```python
from build123d import *

# Parameters (mm, degrees)
BOSS_EXTRUDE2_DEPTH      = 1
SKETCH5_R                = 0.7
CUT_EXTRUDE2_DEPTH       = 1
LPATTERN2_COUNT          = 18
LPATTERN2_PITCH          = 2.47
MIRROR1_COPY_1_SKETCH_R  = 0.7
MIRROR1_COPY_1_DEPTH     = 1
MIRROR1_COPY_2_SKETCH_R  = 0.7
MIRROR1_COPY_2_DEPTH     = 1
MIRROR1_COPY_3_SKETCH_R  = 0.7
MIRROR1_COPY_3_DEPTH     = 1
MIRROR1_COPY_4_SKETCH_R  = 0.7
MIRROR1_COPY_4_DEPTH     = 1
MIRROR1_COPY_5_SKETCH_R  = 0.7
MIRROR1_COPY_5_DEPTH     = 1
MIRROR1_COPY_6_SKETCH_R  = 0.7
MIRROR1_COPY_6_DEPTH     = 1
MIRROR1_COPY_7_SKETCH_R  = 0.7
MIRROR1_COPY_7_DEPTH     = 1
MIRROR1_COPY_8_SKETCH_R  = 0.7
MIRROR1_COPY_8_DEPTH     = 1
MIRROR1_COPY_9_SKETCH_R  = 0.7
MIRROR1_COPY_9_DEPTH     = 1
MIRROR1_COPY_10_SKETCH_R = 0.7
MIRROR1_COPY_10_DEPTH    = 1
MIRROR1_COPY_11_SKETCH_R = 0.7
MIRROR1_COPY_11_DEPTH    = 1
MIRROR1_COPY_12_SKETCH_R = 0.7
MIRROR1_COPY_12_DEPTH    = 1
MIRROR1_COPY_13_SKETCH_R = 0.7
MIRROR1_COPY_13_DEPTH    = 1
MIRROR1_COPY_14_SKETCH_R = 0.7
MIRROR1_COPY_14_DEPTH    = 1
MIRROR1_COPY_15_SKETCH_R = 0.7
MIRROR1_COPY_15_DEPTH    = 1
MIRROR1_COPY_16_SKETCH_R = 0.7
MIRROR1_COPY_16_DEPTH    = 1
MIRROR1_COPY_17_SKETCH_R = 0.7
MIRROR1_COPY_17_DEPTH    = 1
SKETCH6_W                = 27.254379167
SKETCH6_H                = 15.23216969
BOSS_EXTRUDE3_DEPTH      = 4


with BuildPart() as part:
    # Sketch4 → Boss-Extrude2 (new body)
    with BuildSketch(Plane(origin=(0, 0, 0), x_dir=(1, 0, 0), z_dir=(0, 1, 0))):
        Polygon((-23, -10), (23, -10), (23, -8), (27, -8), (27, 8), (23, 8), (23, 10), (-23, 10), align=None)
    extrude(amount=BOSS_EXTRUDE2_DEPTH)

    # Sketch5 → Cut-Extrude2 (cut)
    with BuildSketch(Plane(origin=(0, 1, 0), x_dir=(1, 0, 0), z_dir=(0, 1, 0))):
        with Locations((-21, 10)):
            Circle(SKETCH5_R)
    cut_extrude2 = extrude(amount=-CUT_EXTRUDE2_DEPTH, mode=Mode.SUBTRACT)

    # LPattern2: Cut-Extrude2 ×18
    with Locations(*[(i * LPATTERN2_PITCH, 0, 0) for i in range(1, LPATTERN2_COUNT)]):
        add(cut_extrude2, mode=Mode.SUBTRACT)

    # Mirror1: Cut-Extrude2 across plane
    add(cut_extrude2.mirror(Plane.XY), mode=Mode.SUBTRACT)

    # Mirror1 copy 1 sketch → Mirror1 copy 1 (cut)
    with BuildSketch(Plane(origin=(2.47, 1, 0), x_dir=(1, 0, 0), z_dir=(0, 1, 0))):
        with Locations((-21, -10)):
            Circle(MIRROR1_COPY_1_SKETCH_R)
    extrude(amount=-MIRROR1_COPY_1_DEPTH, mode=Mode.SUBTRACT)

    # Mirror1 copy 2 sketch → Mirror1 copy 2 (cut)
    with BuildSketch(Plane(origin=(4.94, 1, 0), x_dir=(1, 0, 0), z_dir=(0, 1, 0))):
        with Locations((-21, -10)):
            Circle(MIRROR1_COPY_2_SKETCH_R)
    extrude(amount=-MIRROR1_COPY_2_DEPTH, mode=Mode.SUBTRACT)

    # Mirror1 copy 3 sketch → Mirror1 copy 3 (cut)
    with BuildSketch(Plane(origin=(7.41, 1, 0), x_dir=(1, 0, 0), z_dir=(0, 1, 0))):
        with Locations((-21, -10)):
            Circle(MIRROR1_COPY_3_SKETCH_R)
    extrude(amount=-MIRROR1_COPY_3_DEPTH, mode=Mode.SUBTRACT)

    # Mirror1 copy 4 sketch → Mirror1 copy 4 (cut)
    with BuildSketch(Plane(origin=(9.88, 1, 0), x_dir=(1, 0, 0), z_dir=(0, 1, 0))):
        with Locations((-21, -10)):
            Circle(MIRROR1_COPY_4_SKETCH_R)
    extrude(amount=-MIRROR1_COPY_4_DEPTH, mode=Mode.SUBTRACT)

    # Mirror1 copy 5 sketch → Mirror1 copy 5 (cut)
    with BuildSketch(Plane(origin=(12.35, 1, 0), x_dir=(1, 0, 0), z_dir=(0, 1, 0))):
        with Locations((-21, -10)):
            Circle(MIRROR1_COPY_5_SKETCH_R)
    extrude(amount=-MIRROR1_COPY_5_DEPTH, mode=Mode.SUBTRACT)

    # Mirror1 copy 6 sketch → Mirror1 copy 6 (cut)
    with BuildSketch(Plane(origin=(14.82, 1, 0), x_dir=(1, 0, 0), z_dir=(0, 1, 0))):
        with Locations((-21, -10)):
            Circle(MIRROR1_COPY_6_SKETCH_R)
    extrude(amount=-MIRROR1_COPY_6_DEPTH, mode=Mode.SUBTRACT)

    # Mirror1 copy 7 sketch → Mirror1 copy 7 (cut)
    with BuildSketch(Plane(origin=(17.29, 1, 0), x_dir=(1, 0, 0), z_dir=(0, 1, 0))):
        with Locations((-21, -10)):
            Circle(MIRROR1_COPY_7_SKETCH_R)
    extrude(amount=-MIRROR1_COPY_7_DEPTH, mode=Mode.SUBTRACT)

    # Mirror1 copy 8 sketch → Mirror1 copy 8 (cut)
    with BuildSketch(Plane(origin=(19.76, 1, 0), x_dir=(1, 0, 0), z_dir=(0, 1, 0))):
        with Locations((-21, -10)):
            Circle(MIRROR1_COPY_8_SKETCH_R)
    extrude(amount=-MIRROR1_COPY_8_DEPTH, mode=Mode.SUBTRACT)

    # Mirror1 copy 9 sketch → Mirror1 copy 9 (cut)
    with BuildSketch(Plane(origin=(22.23, 1, 0), x_dir=(1, 0, 0), z_dir=(0, 1, 0))):
        with Locations((-21, -10)):
            Circle(MIRROR1_COPY_9_SKETCH_R)
    extrude(amount=-MIRROR1_COPY_9_DEPTH, mode=Mode.SUBTRACT)

    # Mirror1 copy 10 sketch → Mirror1 copy 10 (cut)
    with BuildSketch(Plane(origin=(24.7, 1, 0), x_dir=(1, 0, 0), z_dir=(0, 1, 0))):
        with Locations((-21, -10)):
            Circle(MIRROR1_COPY_10_SKETCH_R)
    extrude(amount=-MIRROR1_COPY_10_DEPTH, mode=Mode.SUBTRACT)

    # Mirror1 copy 11 sketch → Mirror1 copy 11 (cut)
    with BuildSketch(Plane(origin=(27.17, 1, 0), x_dir=(1, 0, 0), z_dir=(0, 1, 0))):
        with Locations((-21, -10)):
            Circle(MIRROR1_COPY_11_SKETCH_R)
    extrude(amount=-MIRROR1_COPY_11_DEPTH, mode=Mode.SUBTRACT)

    # Mirror1 copy 12 sketch → Mirror1 copy 12 (cut)
    with BuildSketch(Plane(origin=(29.64, 1, 0), x_dir=(1, 0, 0), z_dir=(0, 1, 0))):
        with Locations((-21, -10)):
            Circle(MIRROR1_COPY_12_SKETCH_R)
    extrude(amount=-MIRROR1_COPY_12_DEPTH, mode=Mode.SUBTRACT)

    # Mirror1 copy 13 sketch → Mirror1 copy 13 (cut)
    with BuildSketch(Plane(origin=(32.11, 1, 0), x_dir=(1, 0, 0), z_dir=(0, 1, 0))):
        with Locations((-21, -10)):
            Circle(MIRROR1_COPY_13_SKETCH_R)
    extrude(amount=-MIRROR1_COPY_13_DEPTH, mode=Mode.SUBTRACT)

    # Mirror1 copy 14 sketch → Mirror1 copy 14 (cut)
    with BuildSketch(Plane(origin=(34.58, 1, 0), x_dir=(1, 0, 0), z_dir=(0, 1, 0))):
        with Locations((-21, -10)):
            Circle(MIRROR1_COPY_14_SKETCH_R)
    extrude(amount=-MIRROR1_COPY_14_DEPTH, mode=Mode.SUBTRACT)

    # Mirror1 copy 15 sketch → Mirror1 copy 15 (cut)
    with BuildSketch(Plane(origin=(37.05, 1, 0), x_dir=(1, 0, 0), z_dir=(0, 1, 0))):
        with Locations((-21, -10)):
            Circle(MIRROR1_COPY_15_SKETCH_R)
    extrude(amount=-MIRROR1_COPY_15_DEPTH, mode=Mode.SUBTRACT)

    # Mirror1 copy 16 sketch → Mirror1 copy 16 (cut)
    with BuildSketch(Plane(origin=(39.52, 1, 0), x_dir=(1, 0, 0), z_dir=(0, 1, 0))):
        with Locations((-21, -10)):
            Circle(MIRROR1_COPY_16_SKETCH_R)
    extrude(amount=-MIRROR1_COPY_16_DEPTH, mode=Mode.SUBTRACT)

    # Mirror1 copy 17 sketch → Mirror1 copy 17 (cut)
    with BuildSketch(Plane(origin=(41.99, 1, 0), x_dir=(1, 0, 0), z_dir=(0, 1, 0))):
        with Locations((-21, -10)):
            Circle(MIRROR1_COPY_17_SKETCH_R)
    extrude(amount=-MIRROR1_COPY_17_DEPTH, mode=Mode.SUBTRACT)

    # Sketch6 → Boss-Extrude3 (add)
    with BuildSketch(Plane(origin=(0, 1, 0), x_dir=(1, 0, 0), z_dir=(0, 1, 0))):
        with Locations((-8.447512014, 0)):
            Rectangle(SKETCH6_W, SKETCH6_H)
    extrude(amount=BOSS_EXTRUDE3_DEPTH)


solid = part.part
```
Verification items for the finished model (mm, model axes). A direction names the side the tool comes from. Coordinates: 2 decimals unless noted, no trailing zeros. Write each loop counter-clockwise with the first axis right and the second up, starting at its lowest first coordinate (ties: lowest second). Pieces come first, ordered by that corner, then holes. Notation, with made-up numbers: (71, 61.5) - (128, 61.5) arc R19 cw to (128, 72.5) - close; hole circle Ø4 at (-15.5, 47.25). An arc over 180 degrees is marked (long way). Write item = value, one per line.
Q1. Cross-section at D-D (x = 13.58). Enter the section's corners in (y, z).
Answer:
outline = (0, -9.3) - (1, -9.3) - (1, 9.3) - (0, 9.3) - close
Q2. Material ranges on L1, parallel to Y at x = 20.5, z = 9; L2, parallel to X at y = 2.25, z = -1; L3, parallel to Z at x = -1, y = 2.35, recorded low to high. Write a range as from..to.
Answer:
L1 = 0..1
L2 = -22.07..5.18
L3 = -7.62..7.62
Q3. Cross-section at A-A (z = 5.5). Enter the section's corners in (x, y).
Answer:
outline = (-23, 0) - (27, 0) - (27, 1) - (5.18, 1) - (5.18, 5) - (-22.07, 5) - (-22.07, 1) - (-23, 1) - close
Q4. Mould release check, pull along X, two halves, no side actions. Record for faces 4 (the face through (13.6, 0.5, -9.3)), 5 (the face through (0, 0.5, 10)), 6 (the face through (23, 0.5, -9)), 7 (the face through (16.1, 0.5, 9.3)): released by +X, released by -X, zero draft, split by the parting line, or undercut.
Answer:
face_4 = undercut
face_5 = zero draft
face_6 = released by +X
face_7 = undercut
Q5. Cross-section at C-C (y = 2.85). Enter the section's corners in (x, z).
Answer:
outline = (-22.07, -7.62) - (5.18, -7.62) - (5.18, 7.62) - (-22.07, 7.62) - close
Q6. Cross-section at B-B (x = -21). Enter the section's corners in (y, z).
Answer:
outline = (0, -9.3) - (1, -9.3) - (1, -7.62) - (5, -7.62) - (5, 7.62) - (1, 7.62) - (1, 9.3) - (0, 9.3) - close
Q7. Access from +Z, -Z, +X, -X, +Y, -Y to the whole of each face (thin tool, end or side, straight path). Record for faces 1 (the face through (-9, 3, -7.616)), 2 (the face through (-9, 3, 7.616)), 3 (the face through (17.3, 0.5, -10)).
Answer:
face_1 = -Z, +X, -X, +Y
face_2 = +Z, +X, -X, +Y
face_3 = -Z, +X, -X, +Y, -Y
Q8. Go/stop test with flat-tipped pins: pin 1 Ø0.5 at (x, y) = (24.5, 0.5) entering from +Z; pin 2 Ø2 at (y, z) = (3, -7) entering from +X; pin 3 Ø2 at (y, z) = (1.5, -2.5) entering from -X; pin 4 Ø1.2 at (x, y) = (-9, 2.5) entering from -Z. Record where each tip stops, or that it passes through.
Answer:
pin_1 = 8
pin_2 = 5.18
pin_3 = -23
pin_4 = -7.62
